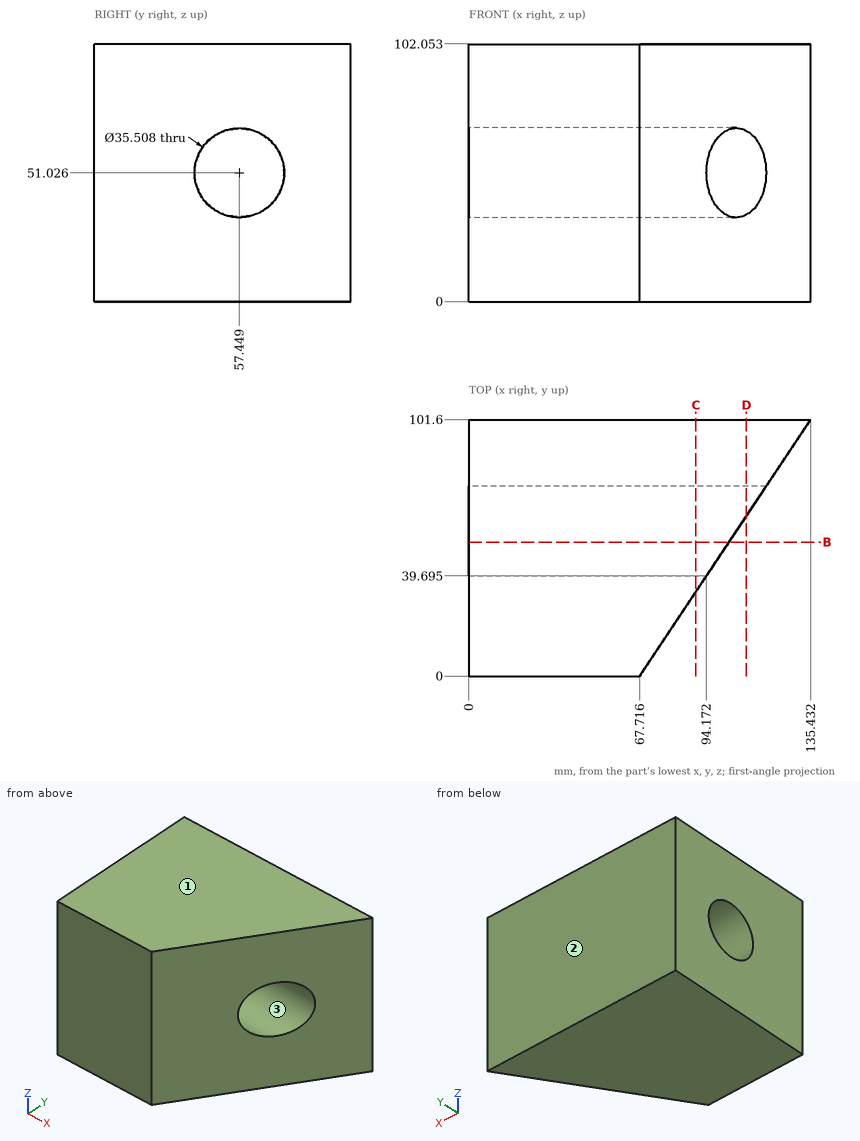
Geometry: see drawing. Coordinates: mm, zero at the bounding-box minimum. Give positions to 0.01 mm unless a question says otherwise; leave off trailing zeros. Loops run counter-clockwise (first coordinate to the right, second up) from the corner with the lowest first, then second, coordinate; pieces in that order, holes last. Notation, with made-up numbers: (40, 39) -> (60, 39) arc R21 ccw to (60, 56) -> close; hole circle Ø3 at (40.5, -19.75). An arc over 180 degrees is marked (long way). Use one line per item in the form item = value.
Item 1: Draft query along Y for the marked faces 1, 2 and 3. Return one class per face: pulls with the +Y half, pulls with the -Y half, needs draft (parallel to the pull), parting line crosses it, or undercut.
A:
face_1 = needs draft
face_2 = pulls with the +Y half
face_3 = undercut
Item 2: Section query B-B on y = 53. Output: boundary loops of the cut face in (x, z).
A:
outline = (0, 0) -> (103.04, 0) -> (103.04, 33.84) -> (0, 33.84) -> close; (0, 68.21) -> (103.04, 68.21) -> (103.04, 102.05) -> (0, 102.05) -> close
Item 3: Section query C-C on x = 90. Output: boundary loops of the cut face in (y, z) (1 decimal), and give its area (3 significant figures).
A:
outline = (33.4, 0) -> (101.6, 0) -> (101.6, 102.1) -> (33.4, 102.1) -> close; hole circle Ø35.5 at (57.4, 51)
area = 5,970 mm^2
Item 4: Section query D-D on x = 110. Output: boundary loops of the cut face in (y, z) (1 decimal).
A:
outline = (63.4, 0) -> (101.6, 0) -> (101.6, 102.1) -> (63.4, 102.1) -> (63.4, 67.7) arc R17.8 cw to (63.4, 34.3) -> close
Item 5: Line query: probe 1 along Y at (x, z) = (8, 50.5) (1 decimal); probe 2 along Z at (x, y) = (38.5, 57.5); probe 3 along Y at (x, z) = (27, 53.5). Output: solid intervals per line, ascending.
A:
probe_1 = 0 to 39.7, 75.2 to 101.6
probe_2 = 0 to 33.27, 68.78 to 102.05
probe_3 = 0 to 39.87, 75.03 to 101.6
